The listing builds one solid part. Answer for the finished solid, in the listing's coordinates (mm). A direction names the side the tool comes from. Give positions to 0.01 mm unless a question says otherwise; leave off trailing zeros. Write each loop counter-clockwise with the first axis right and the second up, starting at its lowest first coordinate (ties: lowest second). Pieces come first, ordered by that corner, then holes. Notation, with made-up numbers: (-1.75, 42) - (20.25, 42) arc R29 ccw to (20.25, 74) - close; hole circle Ø6 at (62.25, 69). An arc over 180 degrees is marked (long way). One line per question, with ' | ' between items. Start each with the question number.
1. A cutting plane is placed at A-A (x = 99). Determine the outline of the cut face in (y, z), then the cut area to 3 significant figures.
2. The mould has two halves that part along Y. Classify faces 4 (the face through (101.48, 0.51, -0.33)), 5 (the face through (55, 0, 2)), 6 (the face through (2.97, 8.73, 97.56)): +Y half, -Y half, draft (parallel to the pull), parting line (faces both ways), or undercut.
3. A cutting plane is placed at C-C (z = -37.5). Determine the outline of the cut face in (x, y).
4. For faces 1 (the face through (5, 10, -102)), 2 (the face through (0, 11, 2)), 3 (the face through (2.97, 8.73, -102.44)), determine the directions among +Z, -Z, +X, -X, +Y, -Y from which every point of the face is accessible in a straight line to the end or side of a thin tool.
5. A cutting plane is placed at D-D (x = 20). Determine the outline of the cut face in (y, z), then the cut area to 3 significant figures.
6. A cutting plane is placed at B-B (z = 90). Determine the outline of the cut face in (x, y).
7. Find the intervals of material crossed by L1, parallel to X at y = 17.25, z = 37; L2, parallel to X at y = 0.2, z = -90, in increasing order. Write a range as from..to.
8. Given P1, Ø8, axis at x = 99, z = -90, coming from the +Y side; P2, Ø3, axis at y = 10.5, z = 19, coming from the -X side; P3, Ø5.5, axis at y = 10, z = -100, coming from the +X side; P4, Ø1.5, axis at y = 13.5, z = -47, coming from the +X side, each flat-ended and moving along its own axis, determine where each tip first touches the part or whether it passes through.
```python
from build123d import *

# Parameters (mm, degrees)
SM_BASE_FLANGE_1_DEPTH = 122.5
CUT_EXTRUDE_1_REACH    = 167.732
SKETCH_4_R             = 2.5
SKETCH_7_R             = 2.75
EXTRUDE_1_DEPTH        = 5
HOLE_WIZARD_M4_1_D     = 3.3
HOLE_WIZARD_M4_1_DEPTH = 10.1
HOLE_WIZARD_M4_1_TIP   = 0.991420021


# Sheet-metal steps are written as plain solids
with BuildPart() as part:
    # Sketch 1 → 基体-法兰1 (new, symmetric)
    with BuildSketch(Plane.XY):
        with BuildLine():
            Line((0, 20), (0, 1.5))
            ThreePointArc((0, 1.5), (0.439339828, 0.439339828), (1.5, 0))
            Line((1.5, 0), (110, 0))
            Line((110, 0), (110, 1))
            Line((110, 1), (1.5, 1))
            ThreePointArc((1.5, 1), (1.146446609, 1.146446609), (1, 1.5))
            Line((1, 1.5), (1, 20))
            Line((1, 20), (0, 20))
        make_face()
    extrude(amount=SM_BASE_FLANGE_1_DEPTH, both=True)

    # 草图4 → 切除-拉伸1 (cut, up to next)
    with BuildSketch(Plane(origin=(0, 1, 0), x_dir=(1, 0, 0), z_dir=(0, 1, 0)), mode=Mode.PRIVATE) as cut_extrude_1_sk1:
        with Locations(Location((99, 0, 0), (0, 0, 270))):
            Circle(SKETCH_4_R)
    cut_extrude_1_tool1 = extrude(cut_extrude_1_sk1.sketch, amount=-CUT_EXTRUDE_1_REACH, mode=Mode.PRIVATE) & part.part
    # 草图4 → 切除-拉伸1 (cut, up to next)
    with BuildSketch(Plane(origin=(0, 1, 0), x_dir=(1, 0, 0), z_dir=(0, 1, 0)), mode=Mode.PRIVATE) as cut_extrude_1_sk2:
        with Locations(Location((99, 90, 0), (0, 0, 270))):
            Circle(SKETCH_4_R)
    cut_extrude_1_tool2 = extrude(cut_extrude_1_sk2.sketch, amount=-CUT_EXTRUDE_1_REACH, mode=Mode.PRIVATE) & part.part
    # 草图4 → 切除-拉伸1 (cut, up to next)
    with BuildSketch(Plane(origin=(0, 1, 0), x_dir=(1, 0, 0), z_dir=(0, 1, 0)), mode=Mode.PRIVATE) as cut_extrude_1_sk3:
        with Locations(Location((99, -90, 0), (0, 0, 270))):
            Circle(SKETCH_4_R)
    cut_extrude_1_tool3 = extrude(cut_extrude_1_sk3.sketch, amount=-CUT_EXTRUDE_1_REACH, mode=Mode.PRIVATE) & part.part
    add(cut_extrude_1_tool1.solids().sort_by_distance((99, 1, 0))[0], mode=Mode.SUBTRACT)
    add(cut_extrude_1_tool2.solids().sort_by_distance((99, 1, -90))[0], mode=Mode.SUBTRACT)
    add(cut_extrude_1_tool3.solids().sort_by_distance((99, 1, 90))[0], mode=Mode.SUBTRACT)

    # 草图7 → 凸台-拉伸1 (add)
    with BuildSketch(Plane.ZY):
        with Locations(Location((0, 10, 0), (0, 0, 270))):
            Circle(SKETCH_7_R)
        with Locations(Location((-100, 10, 0), (0, 0, 270))):
            Circle(SKETCH_7_R)
        with Locations(Location((100, 10, 0), (0, 0, 270))):
            Circle(SKETCH_7_R)
    extrude(amount=-EXTRUDE_1_DEPTH)

    # M4 螺纹孔1
    with Locations(Plane.ZY):
        with Locations((100, 10), (0, 10), (-100, 10)):
            Hole(HOLE_WIZARD_M4_1_D / 2, depth=HOLE_WIZARD_M4_1_DEPTH)
            with Locations((0, 0, -(HOLE_WIZARD_M4_1_DEPTH + HOLE_WIZARD_M4_1_TIP / 2))):  # 118° drill point
                Cone(0, HOLE_WIZARD_M4_1_D / 2, HOLE_WIZARD_M4_1_TIP, mode=Mode.SUBTRACT)


solid = part.part
```
Determined:
1) outline: (0, -122.5) - (1, -122.5) - (1, -92.5) - (0, -92.5) - close; (0, -87.5) - (1, -87.5) - (1, -2.5) - (0, -2.5) - close; (0, 2.5) - (1, 2.5) - (1, 87.5) - (0, 87.5) - close; (0, 92.5) - (1, 92.5) - (1, 122.5) - (0, 122.5) - close | area: 230 mm2
2) face 4: draft | face 5: -Y half | face 6: undercut
3) outline: (0, 1.5) arc R1.5 ccw to (1.5, 0) - (110, 0) - (110, 1) - (1.5, 1) arc R0.5 cw to (1, 1.5) - (1, 20) - (0, 20) - close
4) face 1: +Z, -Z, +X, +Y | face 2: +Z, -Z, -X, +Y, -Y | face 3: +X
5) outline: (0, -122.5) - (1, -122.5) - (1, 122.5) - (0, 122.5) - close | area: 245 mm2
6) outline: (0, 1.5) arc R1.5 ccw to (1.5, 0) - (96.5, 0) - (96.5, 1) - (1.5, 1) arc R0.5 cw to (1, 1.5) - (1, 20) - (0, 20) - close; (101.5, 0) - (110, 0) - (110, 1) - (101.5, 1) - close
7) L1: 0..1 | L2: 0.75..96.5, 101.5..110
8) P1: y = 1 | P2: x = 0 | P3: x = 5 | P4: x = 1
